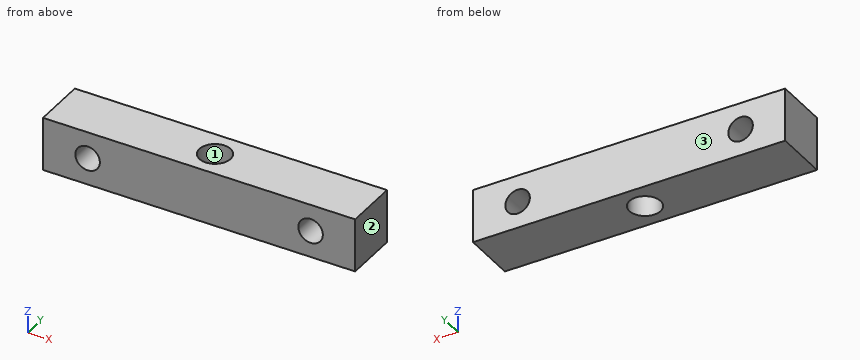
from build123d import *

# Parameters (mm, degrees)
SKETCH1_W                  = 70
SKETCH1_H                  = 12
BOSS_EXTRUDE1_DEPTH        = 12
M8X1_0_TAPPED_HOLE1_D      = 7
F_5_5_5_5_DIAMETER_HOLE1_D = 5.5


with BuildPart() as part:
    # Sketch1 → Boss-Extrude1 (new body)
    with BuildSketch(Plane(origin=(0, 0, 0), x_dir=(1, 0, 0), z_dir=(0, 1, 0))):
        with Locations((35, 6)):
            Rectangle(SKETCH1_W, SKETCH1_H)
    extrude(amount=BOSS_EXTRUDE1_DEPTH)

    # M8x1.0 Tapped Hole1 (through all)
    with Locations(Plane.XY):
        with Locations((35, 6)):
            Hole(M8X1_0_TAPPED_HOLE1_D / 2)

    # Ø5.5 (5.5) Diameter Hole1 (through all)
    with Locations(Plane(origin=(0, 12, 0), x_dir=(-1, 0, 0), z_dir=(0, 1, 0))):
        with Locations((-10, -6), (-60, -6)):
            Hole(F_5_5_5_5_DIAMETER_HOLE1_D / 2)


solid = part.part
Geometry check sheet. Reference: the model listing, model coordinates, mm. Face numbers are marked on the shaded views. Round coordinates to 2 decimals unless told otherwise and drop trailing zeros. Write each loop counter-clockwise with the first axis right and the second up, starting at its lowest first coordinate (ties: lowest second). Pieces come first, ordered by that corner, then holes.
Item 1: Section check C-C (z = -6). Record the boundary of the cut face in (x, y).
Determined:
outline: (0, 0) - (7.25, 0) - (7.25, 12) - (0, 12) - close; (12.75, 0) - (57.25, 0) - (57.25, 12) - (12.75, 12) - close; (62.75, 0) - (70, 0) - (70, 12) - (62.75, 12) - close; hole circle Ø7 at (35, 6)
Item 2: Section check A-A (y = 6). Record the boundary of the cut face in (x, z), plus the area to 3 significant figures.
Determined:
outline: (0, -12) - (31.5, -12) - (31.5, 0) - (0, 0) - close; (38.5, -12) - (70, -12) - (70, 0) - (38.5, 0) - close; hole circle Ø5.5 at (10, -6); hole circle Ø5.5 at (60, -6)
area: 708 mm2
Item 3: Section check D-D (x = 35). Record the boundary of the cut face in (y, z).
Determined:
outline: (0, -12) - (2.5, -12) - (2.5, 0) - (0, 0) - close; (9.5, -12) - (12, -12) - (12, 0) - (9.5, 0) - close
Item 4: Go/stop test with a flat-tipped pin: pin 1 Ø4 at (x, y) = (46, 10.5) entering from +Z. Record where the tip stops, or that it passes through.
Determined:
pin 1: stops at z = 0
Item 5: Mould release check, pull along X, two halves, no side actions. Record for the marked faces 1, 2 and 3: +X half, -X half, draft (parallel to the pull), parting line (faces both ways), or undercut.
Determined:
face 1: undercut
face 2: +X half
face 3: draft
Item 6: Material ranges on line 1 along Z through (x, y) = (60, 5.5); line 2 along X through (y, z) = (1.25, -8); line 3 along X through (y, z) = (2, -8.25), recorded low to high.
Determined:
line 1: z = -12 to -8.75, -3.25 to 0
line 2: x = 0 to 8.11, 11.89 to 58.11, 61.89 to 70
line 3: x = 0 to 8.42, 11.58 to 58.42, 61.58 to 70
Item 7: Section check B-B (x = 60). Record the boundary of the cut face in (y, z), plus the area to 3 significant figures.
Determined:
outline: (0, -12) - (12, -12) - (12, -8.75) - (0, -8.75) - close; (0, -3.25) - (12, -3.25) - (12, 0) - (0, 0) - close
area: 78.0 mm2
